```python
from build123d import *

# Parameters (mm, degrees)
F1_DEPTH = 9
F3_DEPTH = 21


with BuildPart() as f1:
    # F0 (on Top) → F1 (new body)
    with BuildSketch(Plane.XY):
        with BuildLine():
            Line((-51, 0), (0, 0))
            Line((0, 0), (9, 9))
            Line((9, 9), (9, 21))
            Line((9, 21), (0, 30))
            Line((0, 30), (-51, 30))
            ThreePointArc((-51, 30), (-66, 15), (-51, 0))
        make_face()
    extrude(amount=F1_DEPTH)

    # F2 (on face) → F3 (join)
    with BuildSketch(Plane.XY.offset(9)):
        with BuildLine():
            Line((-33, 18.583739), (-33, 30))
            Line((-33, 30), (-51, 30))
            ThreePointArc((-51, 30), (-66, 15), (-51, 0))
            Line((-51, 0), (-33, 0))
            Line((-33, 0), (-33, 11.583739))
            Line((-33, 11.583739), (9, 11.583739))
            Line((9, 11.583739), (9, 18.583739))
            Line((9, 18.583739), (-33, 18.583739))
        make_face()
    extrude(amount=F3_DEPTH)


solid = f1.part
```
Could you check a few things on this model? Use its own coordinates, in mm. A direction names the side the tool comes from. Round coordinates to 2 decimals unless told otherwise and drop trailing zeros. Loops run counter-clockwise (first coordinate to the right, second up) from the corner with the lowest first, then second, coordinate; pieces in that order, holes last. Notation, with made-up numbers: (27, 39) -> (35, 39) arc R30 cw to (35, 70) -> close; hole circle Ø6 at (36, 80.25). An arc over 180 degrees is marked (long way). One line per question, with ' | ' between items.
(1) If I drill on probe 1 along Y at (x, z) = (-27.5, 23.75); probe 2 along Z at (x, y) = (-0.5, 26); probe 3 along X at (y, z) = (24, 11.5), over which ranges is the centre line in solid material (lowest first)?
Model answer:
probe 1: y = 11.58 to 18.58 | probe 2: z = 0 to 9 | probe 3: x = -63 to -33
(2) Thinking about a two-plate mould opening in Y: for faces 1 (the face through (-66, 15, 15)), 2 (the face through (-12, 18.584, 19)), 3 (the face through (-32, 0, 8)), 4 (the face through (-33, 24, 19)), which applies, released by +Y, released by -Y, zero draft, split by the parting line, or undercut?
Model answer:
face 1: split by the parting line | face 2: released by +Y | face 3: released by -Y | face 4: zero draft
(3) If we section it at D-D on y = 4.5: List the corners of the cut face in (x, z) for me.
Model answer:
outline: (-61.71, 0) -> (4.5, 0) -> (4.5, 9) -> (-33, 9) -> (-33, 30) -> (-61.71, 30) -> close
(4) If we section it at A-A on z = 12: List the corners of the cut face in (x, y) for me, and give its area (3 significant figures).
Model answer:
outline: (-51, 0) -> (-33, 0) -> (-33, 11.58) -> (9, 11.58) -> (9, 18.58) -> (-33, 18.58) -> (-33, 30) -> (-51, 30) arc R15 ccw to start | area: 1,190 mm^2
(5) If we section it at B-B on x = -26: List the corners of the cut face in (y, z) for me, and give its area (3 significant figures).
Model answer:
outline: (0, 0) -> (30, 0) -> (30, 9) -> (18.58, 9) -> (18.58, 30) -> (11.58, 30) -> (11.58, 9) -> (0, 9) -> close | area: 417 mm^2
(6) For pin 1 Ø3 at (y, z) = (20.5, 17) entering from -X; pin 2 Ø17 at (x, z) = (-19.5, 19.5) entering from -Y; pin 3 Ø8 at (y, z) = (7.5, 17.5) entering from -X, each with a flat end and sliding along its axis, tell me the tip position at first contact or that it passes through.
Model answer:
pin 1: stops at x = -65.46 | pin 2: stops at y = 11.58 | pin 3: stops at x = -65.59
(7) If we section it at C-C on y = 9.75: List the corners of the cut face in (x, z) for me, and give its area (3 significant figures).
Model answer:
outline: (-65.05, 0) -> (9, 0) -> (9, 9) -> (-33, 9) -> (-33, 30) -> (-65.05, 30) -> close | area: 1,340 mm^2
(8) For faces 5 (the face through (9, 15, 11)), 6 (the face through (-33, 6, 19)), 7 (the face through (-12, 24, 9)), which set-ups out of +Z, -Z, +X, -X, +Y, -Y let a thin tool reach every point of the face, with its end or its side?
Model answer:
face 5: +Z, -Z, +X, +Y, -Y | face 6: +Z, +X, -Y | face 7: +Z, +X, +Y
